For this review, take the finished solid that the model builds, in its own axes (mm). Face numbers are marked on the shaded views. A direction names the side the tool comes from. Round coordinates to 2 decimals unless told otherwise and drop trailing zeros. Loops run counter-clockwise (first coordinate to the right, second up) from the corner with the lowest first, then second, coordinate; pieces in that order, holes last. Notation, with made-up numbers: M 43,-11 L 98,-11 A14 cw 98,0 Z; hole C -22.5,62 d5. An arc over 180 degrees is marked long. One line per question, with ' | ' between items. Start each with the question number.
1) For pin 1 Ø2 at (y, z) = (-23, -40.5) entering from +X; pin 2 Ø1 at (y, z) = (-21.5, -14) entering from -X; pin 3 Ø4 at (x, z) = (-37.5, -3) entering from -Y, all flat-tipped, find the tip position at first contact; note any pin that passes through.
2) We need section A-A (y = -18.5). Give the boundary of the cut face in (x, z), and give its area (3 significant figures).
3) We need section C-C (z = -46). Give the boundary of the cut face in (x, y), and give its area (3 significant figures).
4) For the marked faces 1 and 2, list the 3-axis set-ups (+Z, -Z, +X, -X, +Y, -Y) from which the entire face can be reached by the end or side of a thin tool; tool diameter is ignored.
5) For probe 1 along Z at (x, y) = (-41.75, -24.5); probe 2 along Z at (x, y) = (-39.25, -20); probe 3 along Y at (x, z) = (-41, -12.5), list the stretches that pass through material, from the lowest coordinate up. Write a range as from..to.
6) We need section B-B (z = -23). Give the boundary of the cut face in (x, y).
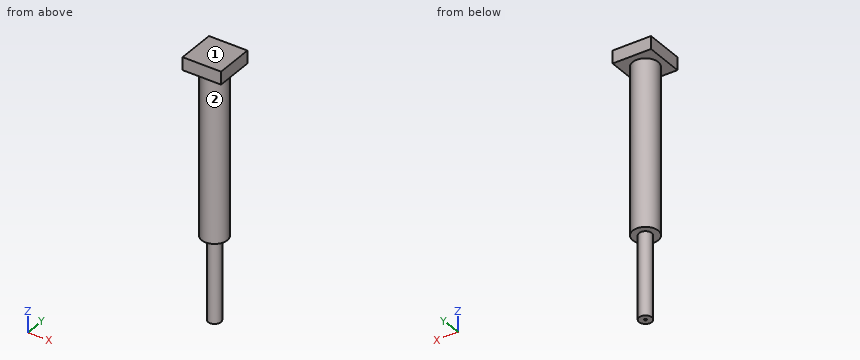
```python
from build123d import *

# Parameters (mm, degrees)
F0_W     = 7.62
F0_H     = 7.62
F1_DEPTH = 2.54
F2_R     = 1.27
F3_DEPTH = 49.53
F4_R     = 0.254
F5_DEPTH = 2.54
F2_R_2   = 2.54
F6_DEPTH = 33.02


with BuildPart() as f1:
    # F0 (on Top) → F1 (new body)
    with BuildSketch(Plane.XY):
        with Locations((-38.795546, -21.835937)):
            Rectangle(F0_W, F0_H)
    extrude(amount=F1_DEPTH)

    # F2 (on face) → F3 (join)
    with BuildSketch(Plane(origin=(0, 0, 0), x_dir=(1, 0, 0), z_dir=(0, 0, -1))):
        with Locations((-38.854431, 21.888208)):
            Circle(F2_R)
    extrude(amount=F3_DEPTH)

    # F4 (on face) → F5 (cut)
    with BuildSketch(Plane(origin=(0, 0, -49.53), x_dir=(1, 0, 0), z_dir=(0, 0, -1))):
        with Locations((-38.854431, 21.888208)):
            Circle(F4_R)
    extrude(amount=-F5_DEPTH, mode=Mode.SUBTRACT)

    # F2 (on face) → F6 (join)
    with BuildSketch(Plane(origin=(0, 0, 0), x_dir=(1, 0, 0), z_dir=(0, 0, -1))):
        with Locations((-38.854431, 21.888208)):
            Circle(F2_R_2)
        with Locations((-38.854431, 21.888208)):
            Circle(F2_R, mode=Mode.SUBTRACT)
    extrude(amount=F6_DEPTH)


solid = f1.part
```
Answers below:
1) pin 1: x = -37.59 | pin 2: x = -41.39 | pin 3: y = -24.43
2) outline: M -42.61,0 L -34.99,0 L -34.99,2.54 L -42.61,2.54 Z | area: 19.4 mm^2
3) outline: C -38.85,-21.89 d2.54 | area: 5.07 mm^2
4) face 1: +Z, +X, -X, +Y, -Y | face 2: -Z
5) probe 1: 0..2.54 | probe 2: -33.02..2.54 | probe 3: -23.25..-20.53
6) outline: C -38.85,-21.89 d5.08
